The model under review builds one solid part; all positions refer to its coordinate system, in mm. A direction names the side the tool comes from. Coordinates: 2 decimals unless noted, no trailing zeros. Write each loop counter-clockwise with the first axis right and the second up, starting at its lowest first coordinate (ties: lowest second). Pieces come first, ordered by that corner, then holes.
```python
from build123d import *

# Parameters (mm, degrees)
BOSS_EXTRUDE1_DEPTH = 3
CUT_EXTRUDE4_START  = -3
SKETCH8_W           = 35
SKETCH8_H           = 65
CUT_EXTRUDE4_DEPTH  = 3
CUT_EXTRUDE5_DEPTH  = 3
CUT_EXTRUDE6_DEPTH  = 3
SKETCH14_W          = 4
SKETCH14_H          = 15
CUT_EXTRUDE7_DEPTH  = 10


with BuildPart() as part:
    # Sketch1 → Boss-Extrude1 (new body)
    with BuildSketch(Plane(origin=(0, 0, 0), x_dir=(1, 0, 0), z_dir=(0, 1, 0))):
        with BuildLine():
            Line((-10, 0), (-115, 0))
            ThreePointArc((-115, 0), (-122.071067812, 2.928932188), (-125, 10))
            Line((-125, 10), (-125, 210))
            ThreePointArc((-125, 210), (-122.071067812, 217.071067812), (-115, 220))
            Line((-115, 220), (-10, 220))
            ThreePointArc((-10, 220), (-2.928932188, 217.071067812), (0, 210))
            Line((0, 210), (0, 10))
            ThreePointArc((0, 10), (-2.928932188, 2.928932188), (-10, 0))
        make_face()
    extrude(amount=BOSS_EXTRUDE1_DEPTH)

    # Sketch8 → Cut-Extrude4 (cut)
    with BuildSketch(Plane(origin=(0, 3, 0), x_dir=(1, 0, 0), z_dir=(0, 1, 0)).offset(CUT_EXTRUDE4_START)):
        with BuildLine():
            Line((-115, 140), (-115, 220))
            ThreePointArc((-115, 220), (-122.071067812, 217.071067812), (-125, 210))
            Line((-125, 210), (-125, 140))
            Line((-125, 140), (-115, 140))
        make_face()
        with Locations((-62.5, 187.5)):
            Rectangle(SKETCH8_W, SKETCH8_H)
        with BuildLine():
            ThreePointArc((0, 210), (-2.928932188, 217.071067812), (-10, 220))
            Line((-10, 220), (-10, 140))
            Line((-10, 140), (0, 140))
            Line((0, 140), (0, 210))
        make_face()
        with BuildLine():
            Line((0, 10), (0, 80))
            Line((0, 80), (-10, 80))
            Line((-10, 80), (-10, 0))
            ThreePointArc((-10, 0), (-2.928932188, 2.928932188), (0, 10))
        make_face()
        with Locations((-62.5, 32.5)):
            Rectangle(SKETCH8_W, SKETCH8_H)
        with BuildLine():
            Line((-115, 80), (-125, 80))
            Line((-125, 80), (-125, 10))
            ThreePointArc((-125, 10), (-122.071067812, 2.928932188), (-115, 0))
            Line((-115, 0), (-115, 80))
        make_face()
    extrude(amount=CUT_EXTRUDE4_DEPTH, mode=Mode.SUBTRACT)

    # Sketch9 → Cut-Extrude5 (cut)
    with BuildSketch(Plane(origin=(0, 3, 0), x_dir=(1, 0, 0), z_dir=(0, 1, 0))):
        Polygon((-81.876757868, 110.403682456), (-71.381014023, 92.224520853), (-50.389526333, 92.224520853), (-39.893782487, 110.403682456), (-50.389526333, 128.582844059), (-71.381014023, 128.582844059), align=None)
    extrude(amount=-CUT_EXTRUDE5_DEPTH, mode=Mode.SUBTRACT)

    # Sketch12 → Cut-Extrude6 (cut)
    with BuildSketch(Plane(origin=(0, 3, 0), x_dir=(1, 0, 0), z_dir=(0, 1, 0))):
        Polygon((-45, 220), (-45, 215), (-40, 220), align=None)
        Polygon((-80, 220), (-85, 220), (-80, 215), align=None)
        Polygon((-115, 215), (-110, 220), (-115, 220), align=None)
        Polygon((0, 140), (-5, 140), (0, 135), align=None)
        Polygon((0, 80), (0, 85), (-5, 80), align=None)
        Polygon((-125, 135), (-120, 140), (-125, 140), align=None)
        Polygon((-110, 0), (-115, 5), (-115, 0), align=None)
        Polygon((-80, 5), (-85, 0), (-80, 0), align=None)
        Polygon((-40, 0), (-45, 5), (-45, 0), align=None)
        Polygon((-10, 0), (-10, 5), (-15, 0), align=None)
        Polygon((-15, 220), (-10, 220), (-10, 215), align=None)
        Polygon((-125, 85), (-120, 80), (-125, 80), align=None)
    extrude(amount=-CUT_EXTRUDE6_DEPTH, mode=Mode.SUBTRACT)

    # Sketch14 → Cut-Extrude7 (cut)
    with BuildSketch(Plane.XZ):
        with Locations((-17.5, -40)):
            Rectangle(SKETCH14_W, SKETCH14_H)
        with Locations((-107.5, -40)):
            Rectangle(SKETCH14_W, SKETCH14_H)
    extrude(amount=-CUT_EXTRUDE7_DEPTH, mode=Mode.SUBTRACT)


solid = part.part
```
Item 1: Take a section at D-D, the plane y = 1.6. Count the separate pieces of the cut face and the enclosed holes in it, plus the area to 3 significant figures.
Solved:
separate pieces: 1
enclosed holes: 3
area: 18,300 mm2
Item 2: Take a section at B-B, the plane z = -200.5. Write out the cut boundary in (x, y), plus the area to 3 significant figures.
Solved:
outline: (-115, 0) - (-80, 0) - (-80, 3) - (-115, 3) - close; (-45, 0) - (-10, 0) - (-10, 3) - (-45, 3) - close
area: 210 mm2
Item 3: For pin 1 (0.9 mm diameter, centred on y = 1.5, z = -180.5, fed in from -X); pin 2 (1.5 mm diameter, centred on x = -117, y = 2, fed in from +Z); pin 3 (1.5 mm diameter, centred on x = -52, y = 1.5, fed in from -Z), all flat-tipped, find the tip position at first contact; note any pin that passes through.
Solved:
pin 1: stops at x = -115
pin 2: stops at z = -80
pin 3: stops at z = -155
Item 4: Machinability: for faces 1 (the face through (-42, 2, -2)), 2 (the face through (-83, 2, -218)), 3 (the face through (-45.07, 1.52, -119.37)), which of the approach directions +Z, -Z, +X, -X, +Y, -Y give a long, thin tool a straight path to every point of the face, cutting with its end or side? Answer none if there is none.
Solved:
face 1: +Z, +Y, -Y
face 2: -Z, +Y, -Y
face 3: +Y, -Y
Item 5: Take a section at C-C, the plane z = -37. Write out the cut boundary in (x, y).
Solved:
outline: (-115, 0) - (-109.5, 0) - (-109.5, 3) - (-115, 3) - close; (-105.5, 0) - (-80, 0) - (-80, 3) - (-105.5, 3) - close; (-45, 0) - (-19.5, 0) - (-19.5, 3) - (-45, 3) - close; (-15.5, 0) - (-10, 0) - (-10, 3) - (-15.5, 3) - close
Item 6: To check wall thickness, follow line 1 along X through (y, z) = (2.45, -35); line 2 along X through (y, z) = (2.2, -203); line 3 along Z through (x, y) = (-63.5, 1.25). State the ranges of each line that lie inside material, in increasing order.
Solved:
line 1: x = -115 to -109.5, -105.5 to -80, -45 to -19.5, -15.5 to -10
line 2: x = -115 to -80, -45 to -10
line 3: z = -155 to -128.58, -92.22 to -65
Item 7: Mouldability with a two-part tool opening along X and no side actions: class faces 4 (the face through (-76.555, 1.521, -119.621)), 5 (the face through (-82, 2, -3)), 6 (the face through (-3, 2, -138)), 7 (the face through (-123, 2, -137)) as pulls with the +X half, pulls with the -X half, needs draft (parallel to the pull), parting line crosses it, or undercut.
Solved:
face 4: undercut
face 5: undercut
face 6: pulls with the +X half
face 7: pulls with the -X half
Item 8: Take a section at A-A, the plane x = -53.5. Write out the cut boundary in (y, z), plus the area to 3 significant figures.
Solved:
outline: (0, -155) - (3, -155) - (3, -128.58) - (0, -128.58) - close; (0, -92.22) - (3, -92.22) - (3, -65) - (0, -65) - close
area: 161 mm2
